For this review, take the finished solid that the model builds, in its own axes (mm). A direction names the side the tool comes from. Give positions to 0.01 mm unless a question says otherwise; leave off trailing zeros. Loops run counter-clockwise (first coordinate to the right, second up) from the corner with the lowest first, then second, coordinate; pieces in that order, holes last. Notation, with made-up numbers: (9.5, 41.5) - (63.5, 41.5) arc R30 cw to (63.5, 73.5) - close; hole circle Ø2 at (-14.5, -22). An arc over 180 degrees is marked (long way). Put each result on its own line as item: value.
from build123d import *

# Parameters (mm, degrees)
SKETCH1_W           = 31.8
SKETCH1_H           = 15.8
BOSS_EXTRUDE1_DEPTH = 9.6
SKETCH2_R           = 2.4
BOSS_EXTRUDE2_DEPTH = 1.8
CUT_EXTRUDE1_START  = 0.7
SKETCH3_R           = 1.3
CUT_EXTRUDE1_DEPTH  = 20.7
SKETCH4_R           = 2.05
SKETCH4_R_2         = 3.25
CUT_EXTRUDE3_DEPTH  = 8.6
CUT_EXTRUDE4_DEPTH  = 2.3


with BuildPart() as part:
    # Sketch1 → Boss-Extrude1 (new body)
    with BuildSketch(Plane.XY):
        Rectangle(SKETCH1_W, SKETCH1_H)
    extrude(amount=BOSS_EXTRUDE1_DEPTH)

    # Sketch2 → Boss-Extrude2 (add)
    with BuildSketch(Plane.XY.offset(9.6)):
        with Locations(Location((-11.9, 3.9, 0), (0, 0, 180))):
            Circle(SKETCH2_R)
        with Locations(Location((-3.9, 3.9, 0), (0, 0, 180))):
            Circle(SKETCH2_R)
        with Locations(Location((4.1, 3.9, 0), (0, 0, 180))):
            Circle(SKETCH2_R)
        with Locations(Location((12.1, 3.9, 0), (0, 0, 180))):
            Circle(SKETCH2_R)
        with Locations(Location((-3.9, -4.1, 0), (0, 0, 180))):
            Circle(SKETCH2_R)
        with Locations(Location((4.1, -4.1, 0), (0, 0, 180))):
            Circle(SKETCH2_R)
        with Locations(Location((12.1, -4.1, 0), (0, 0, 180))):
            Circle(SKETCH2_R)
        with Locations(Location((-11.9, -4.1, 0), (0, 0, 180))):
            Circle(SKETCH2_R)
    extrude(amount=BOSS_EXTRUDE2_DEPTH)

    # Sketch3 → Cut-Extrude1 (cut)
    with BuildSketch(Plane.XY.offset(9.6).offset(CUT_EXTRUDE1_START)):
        with Locations((-11.9, 3.9)):
            Circle(SKETCH3_R)
        with Locations((-3.9, 3.9)):
            Circle(SKETCH3_R)
        with Locations((4.1, 3.9)):
            Circle(SKETCH3_R)
        with Locations((12.1, 3.9)):
            Circle(SKETCH3_R)
        with Locations((-3.9, -4.1)):
            Circle(SKETCH3_R)
        with Locations((4.1, -4.1)):
            Circle(SKETCH3_R)
        with Locations((12.1, -4.1)):
            Circle(SKETCH3_R)
        with Locations((-11.9, -4.1)):
            Circle(SKETCH3_R)
    extrude(amount=-CUT_EXTRUDE1_DEPTH, mode=Mode.SUBTRACT)

    # Sketch4 → Cut-Extrude3 (cut)
    with BuildSketch(Plane.XY):
        with Locations(Location((0, 0, 0), (0, 0, 180))):
            Circle(SKETCH4_R)
        with BuildLine():
            Line((-14.7, 3.4), (-14.7, -3.4))
            Line((-14.7, -3.4), (-14.5, -3.4))
            Line((-14.5, -3.4), (-14.5, -4.6))
            Line((-14.5, -4.6), (-14.7, -4.6))
            Line((-14.7, -4.6), (-14.7, -6.7))
            Line((-14.7, -6.7), (-12.6, -6.7))
            Line((-12.6, -6.7), (-12.6, -6.5))
            Line((-12.6, -6.5), (-11.4, -6.5))
            Line((-11.4, -6.5), (-11.4, -6.7))
            Line((-11.4, -6.7), (-4.6, -6.7))
            Line((-4.6, -6.7), (-4.6, -6.5))
            Line((-4.6, -6.5), (-3.4, -6.5))
            Line((-3.4, -6.5), (-3.4, -6.7))
            Line((-3.4, -6.7), (-0.55, -6.7))
            Line((-0.55, -6.7), (-0.55, -3.203123476))
            ThreePointArc((-0.55, -3.203123476), (-3.25, 0), (-0.55, 3.203123476))
            Line((-0.55, 3.203123476), (-0.55, 6.7))
            Line((-0.55, 6.7), (-3.4, 6.7))
            Line((-3.4, 6.7), (-3.4, 6.5))
            Line((-3.4, 6.5), (-4.6, 6.5))
            Line((-4.6, 6.5), (-4.6, 6.7))
            Line((-4.6, 6.7), (-11.4, 6.7))
            Line((-11.4, 6.7), (-11.4, 6.5))
            Line((-11.4, 6.5), (-12.6, 6.5))
            Line((-12.6, 6.5), (-12.6, 6.7))
            Line((-12.6, 6.7), (-14.7, 6.7))
            Line((-14.7, 6.7), (-14.7, 4.6))
            Line((-14.7, 4.6), (-14.5, 4.6))
            Line((-14.5, 4.6), (-14.5, 3.4))
            Line((-14.5, 3.4), (-14.7, 3.4))
        make_face()
        with Locations(Location((-8, 0, 0), (0, 0, 180))):
            Circle(SKETCH4_R_2, mode=Mode.SUBTRACT)
        with Locations(Location((-8, 0, 0), (0, 0, 180))):
            Circle(SKETCH4_R)
        with BuildLine():
            Line((0.55, -6.7), (0.55, -3.203123476))
            ThreePointArc((0.55, -3.203123476), (3.25, 0), (0.55, 3.203123476))
            Line((0.55, 3.203123476), (0.55, 6.7))
            Line((0.55, 6.7), (3.4, 6.7))
            Line((3.4, 6.7), (3.4, 6.5))
            Line((3.4, 6.5), (4.6, 6.5))
            Line((4.6, 6.5), (4.6, 6.7))
            Line((4.6, 6.7), (11.4, 6.7))
            Line((11.4, 6.7), (11.4, 6.5))
            Line((11.4, 6.5), (12.6, 6.5))
            Line((12.6, 6.5), (12.6, 6.7))
            Line((12.6, 6.7), (14.7, 6.7))
            Line((14.7, 6.7), (14.7, 4.6))
            Line((14.7, 4.6), (14.5, 4.6))
            Line((14.5, 4.6), (14.5, 3.4))
            Line((14.5, 3.4), (14.7, 3.4))
            Line((14.7, 3.4), (14.7, -3.4))
            Line((14.7, -3.4), (14.5, -3.4))
            Line((14.5, -3.4), (14.5, -4.6))
            Line((14.5, -4.6), (14.7, -4.6))
            Line((14.7, -4.6), (14.7, -6.7))
            Line((14.7, -6.7), (12.6, -6.7))
            Line((12.6, -6.7), (12.6, -6.5))
            Line((12.6, -6.5), (11.4, -6.5))
            Line((11.4, -6.5), (11.4, -6.7))
            Line((11.4, -6.7), (4.6, -6.7))
            Line((4.6, -6.7), (4.6, -6.5))
            Line((4.6, -6.5), (3.4, -6.5))
            Line((3.4, -6.5), (3.4, -6.7))
            Line((3.4, -6.7), (0.55, -6.7))
        make_face()
        with Locations(Location((8, 0, 0), (0, 0, 180))):
            Circle(SKETCH4_R_2, mode=Mode.SUBTRACT)
        with Locations(Location((8, 0, 0), (0, 0, 180))):
            Circle(SKETCH4_R)
    extrude(amount=CUT_EXTRUDE3_DEPTH, mode=Mode.SUBTRACT)

    # Sketch5 → Cut-Extrude4 (cut)
    with BuildSketch(Plane.XY):
        with BuildLine():
            Line((0.55, 6.7), (-0.55, 6.7))
            Line((-0.55, 6.7), (-0.55, 3.203123476))
            ThreePointArc((-0.55, 3.203123476), (0, 3.25), (0.55, 3.203123476))
            Line((0.55, 3.203123476), (0.55, 6.7))
        make_face()
        with BuildLine():
            Line((0.55, -6.7), (-0.55, -6.7))
            Line((-0.55, -6.7), (-0.55, -3.203123476))
            ThreePointArc((-0.55, -3.203123476), (0, -3.25), (0.55, -3.203123476))
            Line((0.55, -3.203123476), (0.55, -6.7))
        make_face()
    extrude(amount=CUT_EXTRUDE4_DEPTH, mode=Mode.SUBTRACT)


solid = part.part
1) Insertion check: pin 1 Ø6 at (x, y) = (6, -4) entering from -Z; pin 2 Ø0.8 at (x, y) = (4, -3.5) entering from -Z; pin 3 Ø2 at (x, y) = (4.5, 4) entering from -Z. Each pin has a flat end and moves straight along its axis. Give the tip position at first contact, or say it passes through.
Geometry check:
pin 1: stops at z = 0
pin 2: stops at z = 10.3
pin 3: stops at z = 8.6
2) Wall thickness on line 1 (Y direction, x = 0, z = 2); line 2 (X direction, y = 6, z = 4.25); line 3 (Y direction, x = -14, z = 3.5): over which ranges is each line inside the solid? List them lowest first.
Geometry check:
line 1: y = -7.9 to -6.7, -3.25 to -2.05, 2.05 to 3.25, 6.7 to 7.9
line 2: x = -15.9 to -14.7, -0.55 to 0.55, 14.7 to 15.9
line 3: y = -7.9 to -6.7, 6.7 to 7.9
3) Take a section at D-D on x = -3.9. State the section outline as (y, z) points.
Geometry check:
outline: (-7.9, 0) - (-6.5, 0) - (-6.5, 8.6) - (-5.4, 8.6) - (-5.4, 10.3) - (-2.8, 10.3) - (-2.8, 8.6) - (2.6, 8.6) - (2.6, 10.3) - (5.2, 10.3) - (5.2, 8.6) - (6.5, 8.6) - (6.5, 0) - (7.9, 0) - (7.9, 9.6) - (6.3, 9.6) - (6.3, 11.4) - (1.5, 11.4) - (1.5, 9.6) - (-1.7, 9.6) - (-1.7, 11.4) - (-6.5, 11.4) - (-6.5, 9.6) - (-7.9, 9.6) - close
4) Take a section at C-C on y = 5.5. State the section outline as (x, z) points, and give its area (3 significant figures).
Geometry check:
outline: (-15.9, 0) - (-14.7, 0) - (-14.7, 8.6) - (-0.55, 8.6) - (-0.55, 2.3) - (0.55, 2.3) - (0.55, 8.6) - (14.7, 8.6) - (14.7, 0) - (15.9, 0) - (15.9, 9.6) - (13.89, 9.6) - (13.89, 11.4) - (10.31, 11.4) - (10.31, 9.6) - (5.89, 9.6) - (5.89, 11.4) - (2.31, 11.4) - (2.31, 9.6) - (-2.11, 9.6) - (-2.11, 11.4) - (-5.69, 11.4) - (-5.69, 9.6) - (-10.11, 9.6) - (-10.11, 11.4) - (-13.69, 11.4) - (-13.69, 9.6) - (-15.9, 9.6) - close
area: 85.1 mm²
5) Draft analysis for pull direction Y (two halves, no side actions). For faces 4 (the face through (-15.9, 0, 5)), 5 (the face through (-14.7, 0, 4)), 6 (the face through (-0.55, -5, 5)), state which applies: pulls with the +Y half, pulls with the -Y half, needs draft (parallel to the pull), parting line crosses it, or undercut.
Geometry check:
face 4: needs draft
face 5: undercut
face 6: undercut
6) Take a section at A-A on z = 4.25. State how many separate pieces and enclosed holes the cut face has, and give its area (3 significant figures).
Geometry check:
separate pieces: 3
enclosed holes: 5
area: 179 mm²
7) For faces 1 (the face through (12, -4, 11.4)), 2 (the face through (-6.117, 4.819, 10.487)), 3 (the face through (12, -4, 10.3)), list the 3-axis set-ups (+Z, -Z, +X, -X, +Y, -Y) from which the entire face can be reached by the end or side of a thin tool; tool diameter is ignored.
Geometry check:
face 1: +Z, +X, -X, +Y, -Y
face 2: +Z
face 3: -Z
8) Take a section at B-B on x = 0. State the section outline as (y, z) points, and give its area (3 significant figures).
Geometry check:
outline: (-7.9, 0) - (-6.7, 0) - (-6.7, 2.3) - (-3.25, 2.3) - (-3.25, 0) - (-2.05, 0) - (-2.05, 8.6) - (2.05, 8.6) - (2.05, 0) - (3.25, 0) - (3.25, 2.3) - (6.7, 2.3) - (6.7, 0) - (7.9, 0) - (7.9, 9.6) - (-7.9, 9.6) - close
area: 101 mm²
